Study the drawing (mm; zero at the part's minimum x, y, z) and answer. A direction names the side the tool comes from. Coordinates: 2 decimals unless noted, no trailing zeros. Loops run counter-clockwise (first coordinate to the right, second up) from the corner with the lowest first, then second, coordinate; pieces in that order, holes last.
Q1. Flat-ended cylindrical pins translate along their axes: P1, Ø3, axis at y = 12, z = 5.5, coming from the -X side; P2, Ø2, axis at x = 29, z = 13, coming from the -Y side; P3, Ø4.5, axis at x = 50, z = 8, coming from the -Y side. Find the tip coordinate at first contact, or state that the pin passes through.
Q2. Section D-D (y = 11) is taken. Give the vertices of the cut face in (x, z), then the cut area to 3 significant figures.
Q3. Section A-A (y = 30) is taken. Give the vertices of the cut face in (x, z).
Q4. The mould has two halves that part along X. Classify the marked faces 1, 2 and 3: pulls with the +X half, pulls with the -X half, needs draft (parallel to the pull), parting line crosses it, or undercut.
Q5. Straight lines are drawn through the part: line 1 (X direction, y = 31.5, z = 24.5); line 2 (Y direction, x = 10, z = 6.25); line 3 (X direction, y = 29, z = 7). For each, find the intervals that lie inside material, in ascending order.
Q6. Which of the six approach directions +Z, -Z, +X, -X, +Y, -Y give full straight-line access (tool end or side, diameter ignored) to the marked faces 4, 5 and 6?
Q7. Section C-C (x = 44) is taken. Give the vertices of the cut face in (y, z).
Q8. Section B-B (z = 21) is taken. Give the vertices of the cut face in (x, y), then the cut area to 3 significant figures.
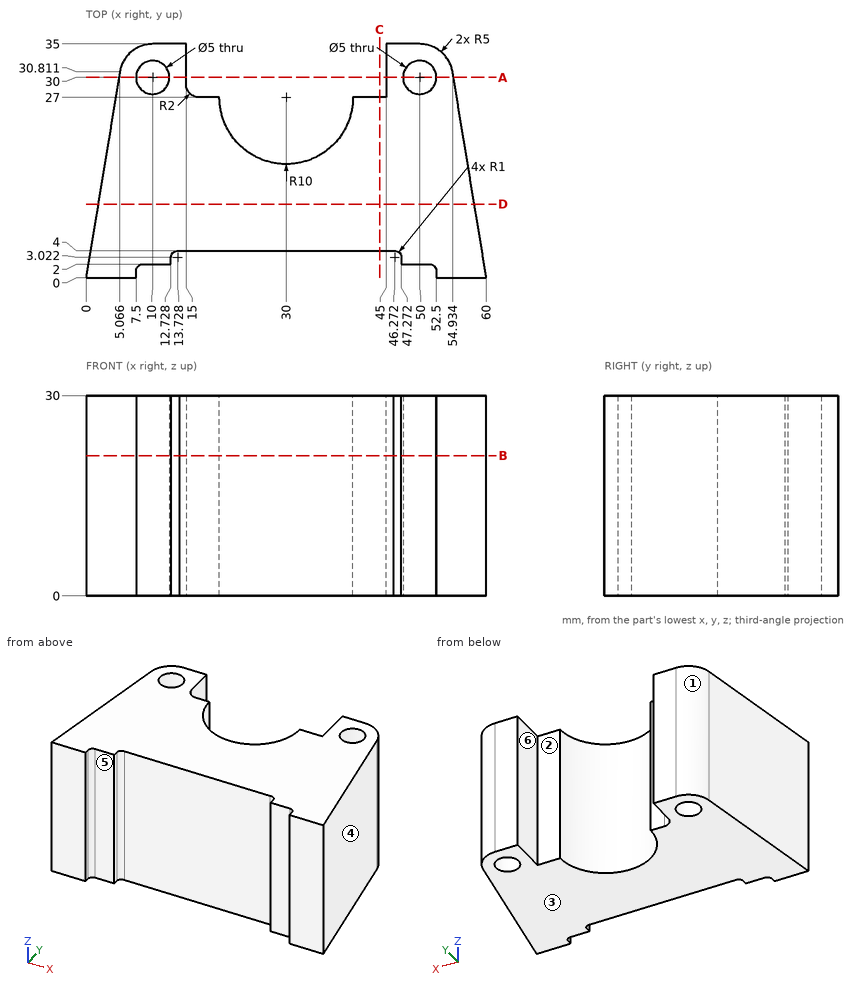
Numbers:
1. P1: stops at x = 1.73
1. P2: stops at y = 4
1. P3: stops at y = 1.66
2. outline: (1.81, 0) - (58.19, 0) - (58.19, 30) - (1.81, 30) - close
2. area: 1,690 mm2
3. outline: (4.93, 0) - (7.5, 0) - (7.5, 30) - (4.93, 30) - close; (12.5, 0) - (15, 0) - (15, 30) - (12.5, 30) - close; (45, 0) - (47.5, 0) - (47.5, 30) - (45, 30) - close; (52.5, 0) - (55.07, 0) - (55.07, 30) - (52.5, 30) - close
4. face 1: pulls with the -X half
4. face 2: undercut
4. face 3: needs draft
5. line 1: x = 5.23 to 8, 12 to 15, 45 to 48, 52 to 54.77
5. line 2: y = 2 to 27.5, 32.5 to 35
5. line 3: x = 4.77 to 7.71, 12.29 to 15, 45 to 47.71, 52.29 to 55.23
6. face 4: +Z, -Z, +X, +Y
6. face 5: +Z, -Z, -Y
6. face 6: +Z, -Z, +Y
7. outline: (4, 0) - (27, 0) - (27, 30) - (4, 30) - close
8. outline: (0, 0) - (7.5, 0) - (7.5, 1) arc R1 cw to (8.5, 2) - (12.73, 2) - (12.73, 3.02) arc R1 cw to (13.94, 4) - (46.06, 4) arc R1 cw to (47.27, 3.02) - (47.27, 2) - (51.5, 2) arc R1 cw to (52.5, 1) - (52.5, 0) - (60, 0) - (54.93, 30.81) arc R5 ccw to (50, 35) - (45, 35) - (45, 27) - (40, 27) arc R10 cw to (20, 27) - (17, 27) arc R2 cw to (15, 29) - (15, 35) - (10, 35) arc R5 ccw to (5.07, 30.81) - close; hole circle Ø5 at (10, 30); hole circle Ø5 at (50, 30)
8. area: 1,300 mm2
